from build123d import *

# Parameters (mm, degrees)
BOSS_EXTRUDE1_DEPTH = 15
FILLET1_R           = 3


with BuildPart() as part:
    # Sketch1 → Boss-Extrude1 (new body)
    with BuildSketch(Plane(origin=(0, 0, 0), x_dir=(1, 0, 0), z_dir=(0, 1, 0))):
        with BuildLine():
            Line((-46.121374994, 46.185937989), (-17.195932558, 11.713938048))
            ThreePointArc((-17.195932558, 11.713938048), (-16.494615838, 6.386908691), (-21.026154773, 3.5))
            Line((-21.026154773, 3.5), (-100, 3.5))
            Line((-100, 3.5), (-100, 0))
            Line((-100, 0), (0, 0))
            Line((0, 0), (0, 6))
            Line((0, 6), (-10.244008888, 18.208334394))
            Line((-10.244008888, 18.208334394), (-12.925164439, 15.958577761))
            Line((-12.925164439, 15.958577761), (-4.568925513, 6))
            Line((-4.568925513, 6), (-7.832443736, 6))
            Line((-7.832443736, 6), (-43.440219443, 48.435694623))
            Line((-43.440219443, 48.435694623), (-46.121374994, 46.185937989))
        make_face()
    extrude(amount=BOSS_EXTRUDE1_DEPTH)

    # Fillet1
    fillet1_edges = [part.edges().sort_by_distance(p)[0] for p in [
        (-10.244008888, 7.5, -18.208334394),
        (-100, 7.5, -3.5),
        (-46.121374994, 7.5, -46.185937989),
    ]]
    fillet(fillet1_edges, radius=FILLET1_R)


solid = part.part
Could you check a few things on this model? Use its own coordinates, in mm. A direction names the side the tool comes from. Coordinates: 2 decimals unless noted, no trailing zeros. Order: outer loops, then holes, each group sorted by start corner. A loop starts at its lowest first (then second) coordinate and runs counter-clockwise, first axis right, second up. Notation, with made-up numbers: (29, 10.5) -> (81, 10.5) arc R34 cw to (81, 47.5) -> close; hole circle Ø11 at (4.25, 17). An arc over 180 degrees is marked (long way). One line per item, written item: value. Start each with the question number.
1) We'd pull the mould along Z, two halves only. Please class faces 1 (the flat face through (-4.1, 7.395, -10.886)), 2 (the cylindrical face through (-16.46, 7.4, -6.46)), 3 (the flat face through (0, 7, -3)): +Z half, -Z half, draft (parallel to the pull), parting line (faces both ways), or undercut.
2) I'm going to push flat-ended pins straight in: pin 1 (2 mm diameter, centred on y = 7.5, z = -36, fed in from -X); pin 2 (3.5 mm diameter, centred on x = -6.5, y = 11, fed in from -Z); pin 3 (1 mm diameter, centred on y = 10.5, z = -39, fed in from +X). Where does each tip first touch, or does it pass through?
3) Imagine slicing it at D-D on x = -66. List the corners of the cut face in (y, z) for me, plus the area to 3 significant figures.
4) Imagine slicing it at B-B on z = -14.5. List the corners of the cut face in (x, y) for me.
5) Which directions (+Z, -Z, +X, -X, +Y, -Y) give clear straight access to the entire face, cutting with the end or side of a thin tool? Please do faces 4 (the cylindrical face through (-10.319, 7.605, -16.967)), 5 (the flat face through (-8.806, 7.395, -11.049)), 6 (the flat face through (-30.883, 7.395, -28.026)).
6) If I drill on L1, parallel to Z at x = -93, y = 11.25; L2, parallel to Z at x = -37.5, y = 5; L3, parallel to Z at x = -23, y = 12.75, over which ranges is the centre line in solid material (lowest first)? Write a range as [from, to].
7) Imagine slicing it at A-A on x = -35.5. List the corners of the cut face in (y, z) for me.
8) Imagine slicing it at C-C on y = 2.75. List the corners of the cut face in (x, z) for me, plus the area to 3 significant figures.
Answer list:
1. face 1: -Z half
1. face 2: undercut
1. face 3: draft
2. pin 1: stops at x = -38.41
2. pin 2: stops at z = -15.83
2. pin 3: stops at x = -35.1
3. outline: (0, -3.5) -> (15, -3.5) -> (15, 0) -> (0, 0) -> close
3. area: 52.5 mm2
4. outline: (-19.53, 0) -> (-14.96, 0) -> (-14.96, 15) -> (-19.53, 15) -> close; (-11.7, 0) -> (-7.13, 0) -> (-7.13, 15) -> (-11.7, 15) -> close
5. face 4: -Z, +Y, -Y
5. face 5: +Y, -Y
5. face 6: -X, +Y, -Y
6. L1: z = [-3.5, 0]
6. L2: z = [-41.36, -35.91], [-3.5, 0]
6. L3: z = [-24.08, -18.63], [-3.5, 0]
7. outline: (0, -38.97) -> (15, -38.97) -> (15, -33.53) -> (0, -33.53) -> close; (0, -3.5) -> (15, -3.5) -> (15, 0) -> (0, 0) -> close
8. outline: (-100, -0.5) arc R3 ccw to (-97, -3.5) -> (-21.03, -3.5) arc R5 cw to (-17.2, -11.71) -> (-44.19, -43.89) arc R3 ccw to (-43.82, -48.11) -> (-43.44, -48.44) -> (-7.83, -6) -> (-4.57, -6) -> (-12.93, -15.96) -> (-12.54, -16.28) arc R3 ccw to (-8.32, -15.91) -> (0, -6) -> (0, 0) -> (-100, 0) -> close
8. area: 637 mm2
